Could you check a few things on this drawing? It's one solid part, dimensions in mm from its lowest x, y, z. Give positions to 0.01 mm unless a question says otherwise; leave off trailing zeros. Order: outer loops, then holes, each group sorted by start corner. A loop starts at its lowest first (then second) coordinate and runs counter-clockwise, first axis right, second up.
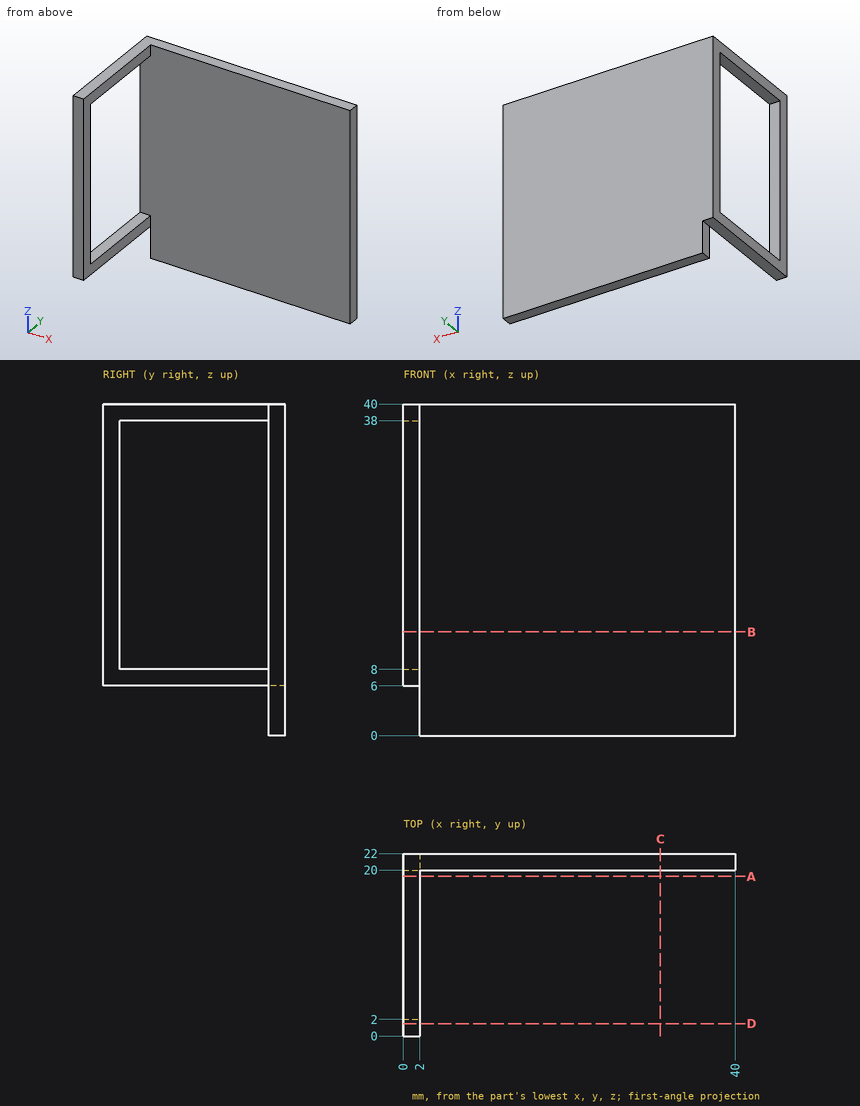
1) I'm going to push flat-ended pins straight in: pin 1 Ø1 at (x, y) = (1, 12.5) entering from -Z; pin 2 Ø2 at (y, z) = (21.5, 3.5) entering from -X; pin 3 Ø6 at (y, z) = (15.5, 25) entering from -X; pin 4 Ø12 at (x, z) = (20, 26.5) entering from -Y. Where does each tip first touch, or does it pass through?
2) Suppose I cut it at B-B (z = 12.5). Please give me the cut outline in (x, y), and give its area (3 significant figures).
3) Suppose I cut it at C-C (x = 31). Please give me the cut outline in (y, z).
4) If I drill on line 1 (Y direction, x = 14.5, z = 10), over which ranges is the centre line in solid material (lowest first)?
5) Suppose I cut it at D-D (y = 1.5). Please give me the cut outline in (x, z).
6) Suppose I cut it at A-A (y = 19.25). Please give me the cut outline in (x, z).
Results:
1. pin 1: stops at z = 6
1. pin 2: stops at x = 2
1. pin 3: passes through
1. pin 4: stops at y = 20
2. outline: (0, 0) - (2, 0) - (2, 2) - (0, 2) - close; (0, 20) - (40, 20) - (40, 22) - (0, 22) - close
2. area: 84.0 mm2
3. outline: (20, 0) - (22, 0) - (22, 40) - (20, 40) - close
4. line 1: y = 20 to 22
5. outline: (0, 6) - (2, 6) - (2, 40) - (0, 40) - close
6. outline: (0, 6) - (2, 6) - (2, 8) - (0, 8) - close; (0, 38) - (2, 38) - (2, 40) - (0, 40) - close
